Part print with two shaded views. Sizes in mm from the minimum x, y, z corner. Give positions to 0.01 mm unless a question says otherwise; leave off trailing zeros. Write each loop counter-clockwise with the first axis right and the second up, starting at its lowest first coordinate (ties: lowest second). Pieces come first, ordered by that corner, then holes. Notation, with made-up numbers: M 66.5,49 L 121.5,49 A35 cw 121.5,86 Z; hole C 51,25 d1. An arc over 180 degrees is marked long. One line per item, written item: value. Start each with the question number.
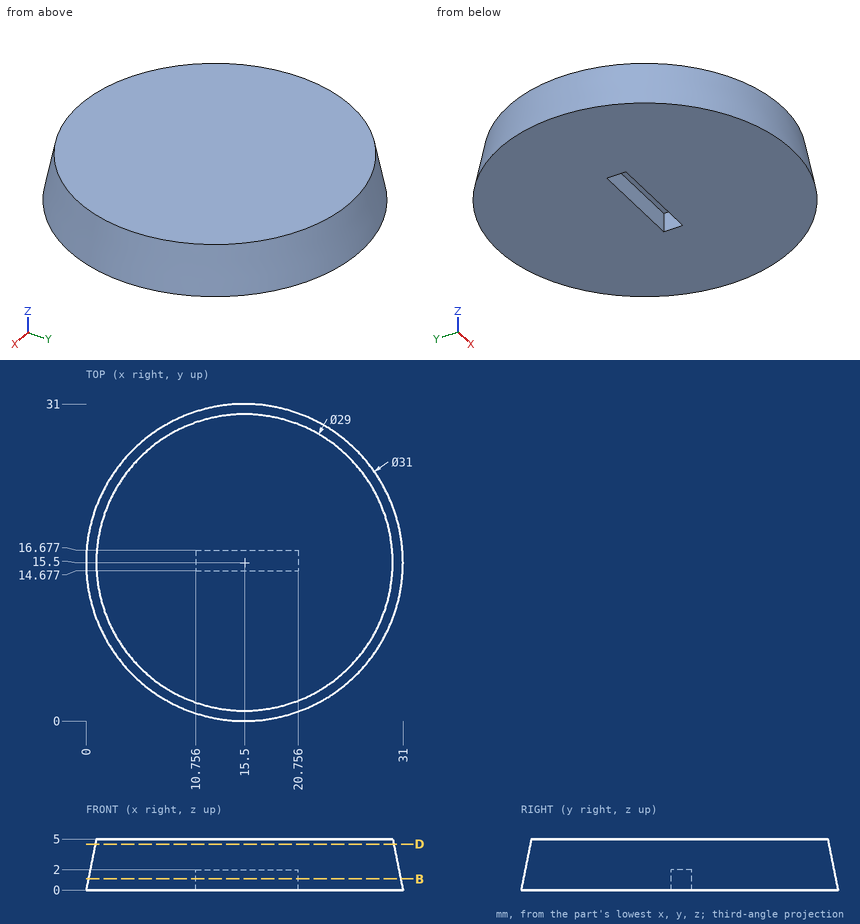
1) Drop flat-ended pins along their axis: P1, Ø0.6, axis at y = 16, z = 0.5, coming from the -X side; P2, Ø6, axis at x = 5, y = 26.5, coming from the -Z side; P3, Ø2, axis at x = 24.5, z = 3.5, coming from the +Y side (1 decimal); P4, Ø1.6, axis at x = 15.5, z = 1, coming from the -Y side. Give the stop position or say it passes through.
2) Probe line 1 along X through (y, z) = (16, 1.3); line 2 along Y through (x, z) = (16.5, 0.95); line 3 along X through (y, z) = (14, 4.6). List the from-to ranges inside material, lowest first. Write a range as from..to.
3) Band-saw the part on D-D (z = 4.5). List the corners of the cut face in (x, y).
4) Band-saw the part on B-B (z = 1.1). List the corners of the cut face in (x, y).
Model answer:
1. P1: stops at x = 0.05
1. P2: stops at z = 0
1. P3: stops at y = 28
1. P4: stops at y = 0.04
2. line 1: x = 0.27..10.76, 20.76..30.73
2. line 2: y = 0.22..14.68, 16.68..30.78
2. line 3: x = 1..30
3. outline: C 15.5,15.5 d29.2
4. outline: C 15.5,15.5 d30.56; hole M 10.76,14.68 L 20.76,14.68 L 20.76,16.68 L 10.76,16.68 Z
